Verification items for the finished model (mm, model axes). Round coordinates to 2 decimals unless told otherwise and drop trailing zeros. Order: outer loops, then holes, each group sorted by start corner. A loop starts at its lowest first (then second) coordinate and runs counter-clockwise, first axis right, second up. Notation, with made-up numbers: M 77.5,44.25 L 85.5,44.25 A21 ccw 85.5,57.25 Z; hole C 70,-13 d5. An arc over 180 degrees is marked long. Use CSV: the item, a comma, the result in double quotes. Start each with the question number.
Q1. Scan lines: line 1 (Z direction, x = -23, y = 0.3); line 2 (Z direction, x = -51, y = 1.75); line 3 (Z direction, x = 69, y = 1.3). Record each from-to range of solid material in increasing order.
Q2. Sectioned sample at B-B (z = 30.5). State how many separate pieces and enclosed holes the cut face has, and give its area (3 significant figures).
Q3. Gauge pin test, flat end, axial feed: pin 1 Ø1 at (x, y) = (-47, 1.5) entering from +Z. Record the tip position at first contact, or that the pin passes through.
Q4. Sectioned sample at A-A (x = -1.5). Enter the section's corners in (y, z).
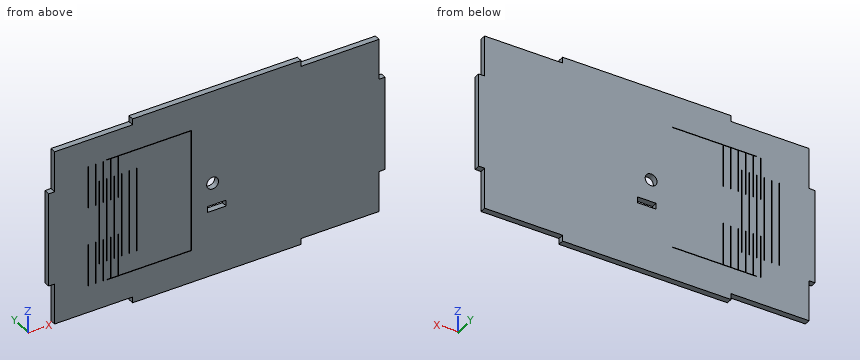
```python
from build123d import *

# Parameters (mm, degrees)
SKETCH1_W                    = 180
SKETCH1_H                    = 100
BOSS_EXTRUDE1_DEPTH          = 3.18
SKETCH3_W                    = 44.91
SKETCH3_H                    = 3.18
CUT_EXTRUDE1_DEPTH           = 3.18
MIRROR2_COPY_1_SKETCH_W      = 44.91
MIRROR2_COPY_1_SKETCH_H      = 3.18
MIRROR2_COPY_1_DEPTH         = 3.18
SKETCH4_W                    = 3.18
SKETCH4_H                    = 24.91
CUT_EXTRUDE2_DEPTH           = 3.18
MIRROR4_COPY_1_SKETCH_W      = 3.18
MIRROR4_COPY_1_SKETCH_H      = 24.91
MIRROR4_COPY_1_DEPTH         = 3.18
SKETCH6_R                    = 3.18
CUT_EXTRUDE3_DEPTH           = 3.18
SKETCH7_W                    = 10
SKETCH7_H                    = 3.18
CUT_EXTRUDE4_DEPTH           = 3.18
SKETCH5_W                    = 0.18
SKETCH5_H                    = 45
SKETCH5_H_2                  = 22.5
CUT_EXTRUDE_THIN1_DEPTH      = 10
LPATTERN2_COUNT              = 5
LPATTERN2_PITCH              = 4
LPATTERN2_COL_COUNT          = 4
LPATTERN2_COL_PITCH          = 4
CUT_EXTRUDE_THIN2_DEPTH      = 1
CUT_EXTRUDE_THIN2_DEPTH_BACK = 10


with BuildPart() as part:
    # Sketch1 → Boss-Extrude1 (new body)
    with BuildSketch(Plane(origin=(0, 0, 0), x_dir=(1, 0, 0), z_dir=(0, 1, 0))):
        Rectangle(SKETCH1_W, SKETCH1_H)
    extrude(amount=BOSS_EXTRUDE1_DEPTH)

    # Sketch3 → Cut-Extrude1 (cut)
    with BuildSketch(Plane(origin=(0, 3.18, 0), x_dir=(1, 0, 0), z_dir=(0, 1, 0))):
        with Locations((67.545, -48.41)):
            Rectangle(SKETCH3_W, SKETCH3_H)
    cut_extrude1 = extrude(amount=-CUT_EXTRUDE1_DEPTH, mode=Mode.SUBTRACT)

    # Mirror1: Cut-Extrude1 across plane
    add(cut_extrude1.mirror(Plane(origin=(0, 0, 0), x_dir=(0, 0, 1), z_dir=(1, 0, 0))), mode=Mode.SUBTRACT)

    # Mirror2: Cut-Extrude1 across plane
    add(cut_extrude1.mirror(Plane.XY), mode=Mode.SUBTRACT)

    # Mirror2 copy 1 sketch → Mirror2 copy 1 (cut)
    with BuildSketch(Plane(origin=(0, 3.18, 0), x_dir=(-1, 0, 0), z_dir=(0, 1, 0))):
        with Locations((67.545, -48.41)):
            Rectangle(MIRROR2_COPY_1_SKETCH_W, MIRROR2_COPY_1_SKETCH_H)
    extrude(amount=-MIRROR2_COPY_1_DEPTH, mode=Mode.SUBTRACT)

    # Sketch4 → Cut-Extrude2 (cut)
    with BuildSketch(Plane(origin=(0, 3.18, 0), x_dir=(1, 0, 0), z_dir=(0, 1, 0))):
        with Locations((-88.41, 37.545)):
            Rectangle(SKETCH4_W, SKETCH4_H)
    cut_extrude2 = extrude(amount=-CUT_EXTRUDE2_DEPTH, mode=Mode.SUBTRACT)

    # Mirror3: Cut-Extrude2 across plane
    add(cut_extrude2.mirror(Plane.XY), mode=Mode.SUBTRACT)

    # Mirror4: Cut-Extrude2 across plane
    add(cut_extrude2.mirror(Plane(origin=(0, 0, 0), x_dir=(0, 0, 1), z_dir=(1, 0, 0))), mode=Mode.SUBTRACT)

    # Mirror4 copy 1 sketch → Mirror4 copy 1 (cut)
    with BuildSketch(Plane(origin=(0, 3.18, 0), x_dir=(-1, 0, 0), z_dir=(0, 1, 0))):
        with Locations((-88.41, 37.545)):
            Rectangle(MIRROR4_COPY_1_SKETCH_W, MIRROR4_COPY_1_SKETCH_H)
    extrude(amount=-MIRROR4_COPY_1_DEPTH, mode=Mode.SUBTRACT)

    # Sketch6 → Cut-Extrude3 (cut)
    with BuildSketch(Plane(origin=(0, 3.18, 0), x_dir=(1, 0, 0), z_dir=(0, 1, 0))):
        with Locations((-2.271207142, 0)):
            Circle(SKETCH6_R)
    extrude(amount=-CUT_EXTRUDE3_DEPTH, mode=Mode.SUBTRACT)

    # Sketch7 → Cut-Extrude4 (cut)
    with BuildSketch(Plane(origin=(0, 3.18, 0), x_dir=(1, 0, 0), z_dir=(0, 1, 0))):
        with Locations((0, 13.41)):
            Rectangle(SKETCH7_W, SKETCH7_H)
    extrude(amount=-CUT_EXTRUDE4_DEPTH, mode=Mode.SUBTRACT)

    # Sketch5 → Cut-Extrude-Thin1 (cut)
    with BuildSketch(Plane(origin=(0, 3.18, 0), x_dir=(1, 0, 0), z_dir=(0, 1, 0))):
        with Locations((-58.861207142, 0)):
            Rectangle(SKETCH5_W, SKETCH5_H)
        with Locations((-56.861207142, 21.25)):
            Rectangle(SKETCH5_W, SKETCH5_H_2)
        with Locations((-56.861207142, -21.25)):
            Rectangle(SKETCH5_W, SKETCH5_H_2)
    cut_extrude_thin1 = extrude(amount=-CUT_EXTRUDE_THIN1_DEPTH, mode=Mode.SUBTRACT)

    # LPattern2: Cut-Extrude-Thin1 ×5
    with Locations(*[(i * LPATTERN2_PITCH, 0, 0) for i in range(1, LPATTERN2_COUNT)]):
        add(cut_extrude_thin1, mode=Mode.SUBTRACT)

    # LPattern2 col: Cut-Extrude-Thin1 ×4
    with Locations(*[(-i * LPATTERN2_COL_PITCH, 0, 0) for i in range(1, LPATTERN2_COL_COUNT)]):
        add(cut_extrude_thin1, mode=Mode.SUBTRACT)

    # Sketch9 → Cut-Extrude-Thin2 (cut, two sides)
    with BuildSketch(Plane(origin=(0, 3.18, 0), x_dir=(1, 0, 0), z_dir=(0, 1, 0))) as cut_extrude_thin2_sk:
        Polygon((-58.771207142, 32.5), (-13.771207142, 32.5), (-13.771207142, -32.5), (-58.951207142, -32.5), (-58.951207142, -32.68), (-13.591207142, -32.68), (-13.591207142, 32.68), (-58.771207142, 32.68), align=None)
    extrude(amount=CUT_EXTRUDE_THIN2_DEPTH, mode=Mode.SUBTRACT)
    extrude(cut_extrude_thin2_sk.sketch, amount=-CUT_EXTRUDE_THIN2_DEPTH_BACK, mode=Mode.SUBTRACT)


solid = part.part
```
Verdict:
1,line 1,"z = -50 to -32.68, -32.5 to 32.5, 32.68 to 50"
1,line 2,"z = -46.82 to -32.68, -32.5 to 32.5, 32.68 to 46.82"
1,line 3,"z = -46.82 to 46.82"
2,separate pieces,"10"
2,enclosed holes,"0"
2,area,"547 mm²"
3,pin 1,"stops at z = 46.82"
4,outline,"M 0,-50 L 3.18,-50 L 3.18,-15 L 0,-15 Z; M 0,-11.82 L 3.18,-11.82 L 3.18,-3.09 L 0,-3.09 Z; M 0,3.09 L 3.18,3.09 L 3.18,50 L 0,50 Z"
